Source: three-view drawing plus pictorial views. Frame: mm from the lowest corner of the part. A direction names the side the tool comes from. Give positions to 0.01 mm unless a question says otherwise; leave off trailing zeros. Order: outer loops, then holes, each group sorted by start corner. A loop starts at its lowest first (then second) coordinate and runs counter-clockwise, first axis right, second up.
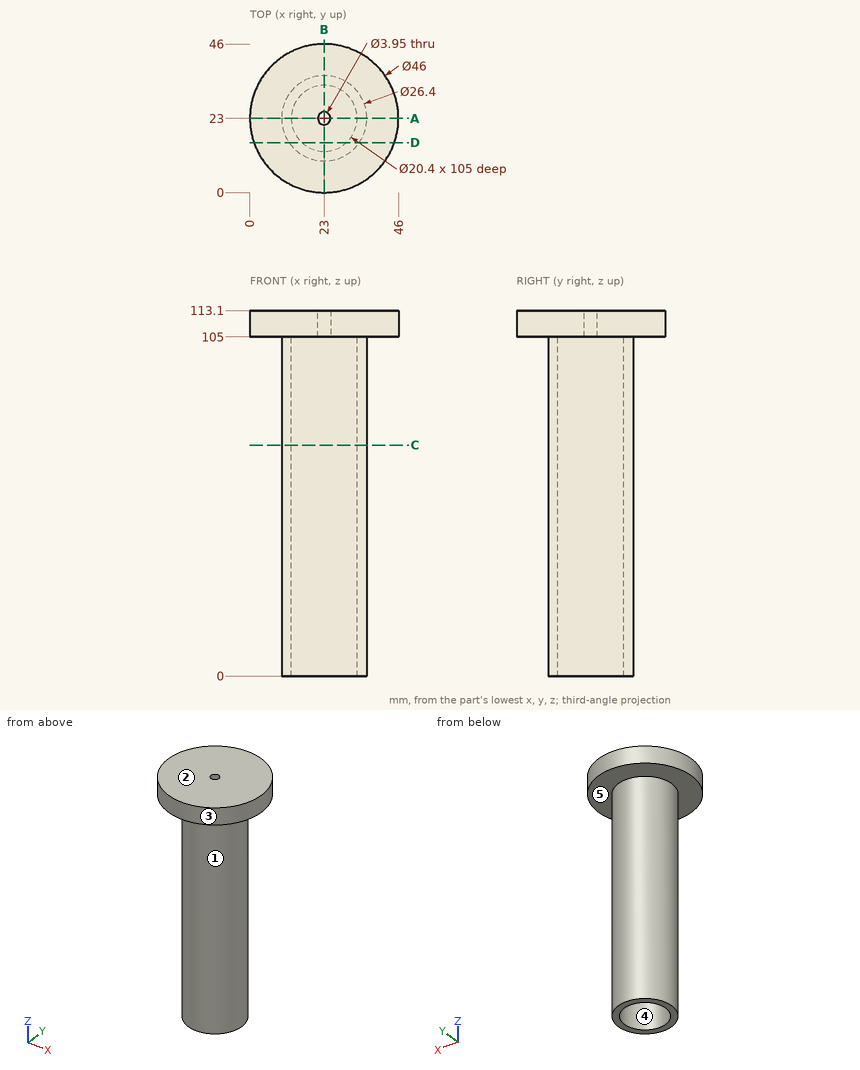
(1) Section D-D, the plane y = 15.5. Return loops of the section in (x, z), plus the area to 3 significant figures.
(2) Section C-C, the plane z = 71.5. Return loops of the section in (x, y), plus the area to 3 significant figures.
(3) Draft query along Y for the marked faces 3, 4 and 5. Return one class per face: +Y half, -Y half, draft (parallel to the pull), parting line (faces both ways), or undercut.
(4) Line query: line 1 along Y through (x, z) = (23, 59); line 2 along Y through (x, z) = (23, 107.75) (3 decimals). Output: solid intervals per line, ascending.
(5) Section A-A, the plane y = 23. Return loops of the section in (x, z) (3 decimals).
(6) Access query for the marked faces 1 and 2. Directions: +Z, -Z, +X, -X, +Y, -Y. A direction counts if a zero-diameter tool reaches every point of the face in a straight line with its end or side. Return the directions, or none.
(7) Pin query (flat end, axial travel): pin 1 Ø10 at (x, z) = (10.5, 59) entering from +Y; pin 2 Ø2 at (x, z) = (26, 29) entering from +Y; pin 3 Ø5 at (x, z) = (16, 28.5) entering from +Y. Return the tip coordinate at first contact, or that it passes through.
Checks:
1. outline: (1.26, 105) - (12.14, 105) - (12.14, 0) - (16.09, 0) - (16.09, 105) - (29.91, 105) - (29.91, 0) - (33.86, 0) - (33.86, 105) - (44.74, 105) - (44.74, 113.1) - (1.26, 113.1) - close
1. area: 1,180 mm2
2. outline: circle Ø26.4 at (23, 23); hole circle Ø20.4 at (23, 23)
2. area: 221 mm2
3. face 3: parting line
3. face 4: undercut
3. face 5: draft
4. line 1: y = 9.8 to 12.8, 33.2 to 36.2
4. line 2: y = 0 to 21.025, 24.975 to 46
5. outline: (0, 105) - (9.8, 105) - (9.8, 0) - (12.8, 0) - (12.8, 105) - (21.025, 105) - (21.025, 113.1) - (0, 113.1) - close; (24.975, 105) - (33.2, 105) - (33.2, 0) - (36.2, 0) - (36.2, 105) - (46, 105) - (46, 113.1) - (24.975, 113.1) - close
6. face 1: -Z
6. face 2: +Z, +X, -X, +Y, -Y
7. pin 1: stops at y = 33.86
7. pin 2: stops at y = 36.05
7. pin 3: stops at y = 35.41
